Input: part model. Units: mm. Frame: model coordinates. A direction names the side the tool comes from. Give positions to 0.01 mm unless a question says otherwise; leave off trailing zeros. Order: outer loops, then holes, each group sorted by start corner. A loop starts at its lowest first (then second) coordinate and runs counter-clockwise, first axis right, second up. Notation, with made-up numbers: (-30.75, -12) - (0.25, -12) arc R34 cw to (0.25, 21) - close; hole circle Ø5 at (-17, 79.5). An arc over 180 degrees is marked (long way). Answer in a Markdown table with one row per item. Add a question column.
1. Section query B-B on x = 2. Return loops of the section in (y, z), and give its area (3 significant figures).
2. Access query for faces 1 (the face through (4, 4.955, -3)), 2 (the face through (4.437, 9.882, -8.003)). Directions: +Z, -Z, +X, -X, +Y, -Y. A direction counts if a zero-diameter tool reaches every point of the face in a straight line with its end or side. Return the directions, or none.
3. Section query D-D on x = 5.75. Return loops of the section in (y, z).
4. Contact query for flat-ended pins moving along their axis: pin 1 (4 mm diameter, centred on x = 4.5, z = -2, fed in from +Y); pin 2 (1.5 mm diameter, centred on x = 1.5, z = -11.5, fed in from -Y); pin 3 (1.5 mm diameter, centred on x = 5, y = 8, fed in from +Z). Output: stop coordinate, or through.
5. Section query A-A on y = 1.5. Return loops of the section in (x, z).
6. Ray query, line 1 (Y direction, x = 2.25, z = -1.5); line 2 (Y direction, x = 6.5, z = -15.75); line 3 (Z direction, x = 7.25, y = 5.5). Return the intervals inside material, ascending. Write a range as [from, to].
7. Section query C-C on z = -4. Return loops of the section in (x, y), and give its area (3 significant figures).
```python
from build123d import *

# Parameters (mm, degrees)
SKETCH_1_W          = 9
SKETCH_1_H          = 24
EXTRUDE_1_DEPTH     = 10
SKETCH_2_W          = 9
SKETCH_2_H          = 5
CUT_EXTRUDE_1_DEPTH = 5.04505
CUT_EXTRUDE_2_DEPTH = 10
CUT_EXTRUDE_4_DEPTH = 11
FILLET_1_R          = 20
FILLET_2_R          = 1
FILLET_3_R          = 2
FILLET_4_R          = 10


with BuildPart() as part:
    # ｽｹｯﾁ1 → ﾎﾞｽ - 押し出し1 (new body)
    with BuildSketch(Plane(origin=(0, 0, 0), x_dir=(1, 0, 0), z_dir=(0, 1, 0))):
        with Locations((4.5, 12)):
            Rectangle(SKETCH_1_W, SKETCH_1_H)
    extrude(amount=EXTRUDE_1_DEPTH)

    # ｽｹｯﾁ2 → ｶｯﾄ - 押し出し1 (cut)
    with BuildSketch(Plane(origin=(0, 10, 0), x_dir=(1, 0, 0), z_dir=(0, 1, 0))):
        with Locations((4.5, 2.5)):
            Rectangle(SKETCH_2_W, SKETCH_2_H)
    extrude(amount=-CUT_EXTRUDE_1_DEPTH, mode=Mode.SUBTRACT)

    # ｽｹｯﾁ3 → ｶｯﾄ - 押し出し2 (cut, through all)
    with BuildSketch(Plane(origin=(9, 0, 0), x_dir=(0, 0, -1), z_dir=(1, 0, 0))):
        Polygon((8, 10), (24, 5), (24, 10), align=None)
        Polygon((10, 0), (24, 0), (24, 2), align=None)
    extrude(amount=-CUT_EXTRUDE_2_DEPTH, mode=Mode.SUBTRACT)

    # ｽｹｯﾁ6 → ｶｯﾄ - 押し出し4 (cut, through all)
    with BuildSketch(Plane.XZ):
        Polygon((9, -24), (9, -17), (6, -24), align=None)
        Polygon((3, -24), (0, -17), (0, -24), align=None)
    extrude(amount=-CUT_EXTRUDE_4_DEPTH, mode=Mode.SUBTRACT)

    # ﾌｨﾚｯﾄ1
    fillet_1_edges = [part.edges().sort_by_distance(p)[0] for p in [
        (4.5, 0, -10),
    ]]
    fillet(fillet_1_edges, radius=FILLET_1_R)

    # ﾌｨﾚｯﾄ2
    fillet_2_edges = [part.edges().sort_by_distance(p)[0] for p in [
        (6, 3.5, -24),
        (3, 3.5, -24),
    ]]
    fillet(fillet_2_edges, radius=FILLET_2_R)

    # ﾌｨﾚｯﾄ3
    fillet_3_edges = [part.edges().sort_by_distance(p)[0] for p in [
        (9, 4.09375, -17),
        (0, 4.09375, -17),
    ]]
    fillet(fillet_3_edges, radius=FILLET_3_R)

    # ﾌｨﾚｯﾄ4
    fillet_4_edges = [part.edges().sort_by_distance(p)[0] for p in [
        (4.5, 10, -8),
    ]]
    fillet(fillet_4_edges, radius=FILLET_4_R)


solid = part.part
```
Answer:
| question | item | result |
|---|---|---|
| 1 | outline | (0, -8.58) arc R20 ccw to (0.2, -11.41) - (1.67, -21.67) - (5.73, -21.67) - (9.54, -9.46) arc R10 ccw to (10, -6.47) - (10, -5) - (4.95, -5) - (4.95, 0) - (0, 0) - close |
| 1 | area | 152 mm² |
| 2 | face 1 | +Z, +X, -X, +Y |
| 2 | face 2 | -Z, +X, -X, +Y |
| 3 | outline | (0, -8.58) arc R20 ccw to (0.2, -11.41) - (1.99, -23.91) - (5.03, -23.91) - (9.54, -9.46) arc R10 ccw to (10, -6.47) - (10, -5) - (4.95, -5) - (4.95, 0) - (0, 0) - close |
| 4 | pin 1 | stops at y = 4.95 |
| 4 | pin 2 | stops at y = 0.12 |
| 4 | pin 3 | stops at z = -5 |
| 5 | outline | (0, -16.59) arc R2 ccw to (0.16, -17.38) - (1.5, -20.5) - (7.5, -20.5) - (8.84, -17.38) arc R2 ccw to (9, -16.59) - (9, 0) - (0, 0) - close |
| 6 | line 1 | y = [0, 4.95] |
| 6 | line 2 | y = [0.82, 7.58] |
| 6 | line 3 | z = [-21.08, -5] |
| 7 | outline | (0, 0) - (9, 0) - (9, 4.95) - (0, 4.95) - close |
| 7 | area | 44.6 mm² |
